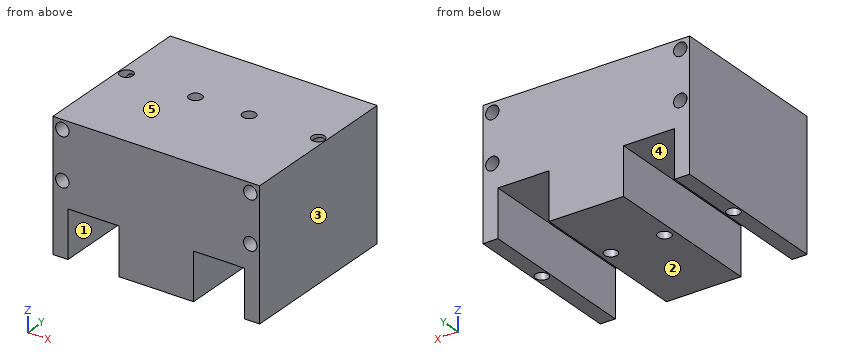
Autodesk Inventor part; units mm, degrees
ref_plane "YZ Plane" through (0, 0, 0) normal (1, 0, 0) x (0, 1, 0)
ref_plane "XZ Plane" through (0, 0, 0) normal (0, 1, 0) x (-1, 0, 0)
ref_plane "XY Plane" through (0, 0, 0) normal (0, 0, 1) x (1, 0, 0)
sketch "Esboço1" plane through (0, 0, 0) normal (0, 1, 0) x (-1, 0, 0)
  line L0 (0, 0) -> (-49.4, 0)
  line L1 (-49.4, 0) -> (-49.4, -15.9)
  line L2 (-49.4, -15.9) -> (0, -15.9)
  line L3 (0, -15.9) -> (0, 0)
  dimension "d0" = 49.4
  dimension "d1" = 15.9
extrude "Extrusão1" add sketch "Esboço1" along normal blind 40
sketch "Esboço2" plane through (0, 40, 0) normal (0, 1, 0) x (1, 0, 0)
  line L0 (49.4, 15.9) -> (0, 15.9)
  line L1 (0, 15.9) -> (4.5, 15.9)
  line L2 (4.5, 15.9) -> (4.5, 11.4)
  line L3 (4.5, 11.4) -> (0, 11.4)
  line L4 (0, 11.4) -> (0, 15.9)
  line L5 (0, 0) -> (49.4, 0)
  line L6 (0, 0) -> (4.5, 0)
  line L7 (4.5, 0) -> (4.5, 4.5)
  line L8 (4.5, 4.5) -> (0, 4.5)
  line L9 (0, 4.5) -> (0, 0)
  line L10 (49.4, 0) -> (49.4, 15.9)
  line L11 (49.4, 15.9) -> (44.9, 15.9)
  line L12 (44.9, 15.9) -> (44.9, 11.4)
  line L13 (44.9, 11.4) -> (49.4, 11.4)
  line L14 (49.4, 11.4) -> (49.4, 15.9)
  line L15 (49.4, 0) -> (44.9, 0)
  line L16 (44.9, 0) -> (44.9, 4.5)
  line L17 (44.9, 4.5) -> (49.4, 4.5)
  line L18 (49.4, 4.5) -> (49.4, 0)
  line L19 (2.25, 15.9) -> (2.25, 11.4)
  line L20 (2.25, 4.5) -> (2.25, 0)
  line L21 (47.15, 15.9) -> (47.15, 11.4)
  line L22 (47.15, 4.5) -> (47.15, 0)
  circle A0 centre (2.25, 13.65) radius 1.6
  circle A1 centre (2.25, 2.25) radius 1.6
  circle A2 centre (47.15, 13.65) radius 1.6
  circle A3 centre (47.15, 2.25) radius 1.6
  dimension "d4" = 4.5
  dimension "d5" = 4.5
  dimension "d6" = 4.5
  dimension "d7" = 4.5
  dimension "d8" = 4.5
  dimension "d9" = 4.5
  dimension "d10" = 4.5
  dimension "d11" = 4.5
  dimension "d12" = 3.2
  dimension "d13" = 3.2
  dimension "d14" = 3.2
  dimension "d15" = 3.2
extrude "Extrusão2" cut sketch "Esboço2" against normal blind 40 contours A2 L21 | L21 A2 | A3 L22 | L22 A3 | A0 L19 | L19 A0 | A1 L20 | L20 A1
sketch "Esboço3" plane through (49.4, 0, -15.9) normal (0, 0, -1) x (-1, 0, 0)
  line L0 (49.4, 40) -> (0, 40)
  line L1 (49.4, 0) -> (33.6, 0)
  line L2 (33.6, 0) -> (33.6, 40)
  line L3 (33.6, 40) -> (49.4, 40)
  line L4 (49.4, 40) -> (49.4, 0)
  line L5 (0, 0) -> (15.8, 0)
  line L6 (15.8, 0) -> (15.8, 40)
  line L7 (15.8, 40) -> (0, 40)
  line L8 (0, 40) -> (0, 0)
  line L9 (33.6, 0) -> (15.8, 0)
  line L10 (15.8, 0) -> (15.8, 40)
  line L11 (15.8, 40) -> (33.6, 40)
  line L12 (33.6, 40) -> (33.6, 0)
  line L13 (49.4, 0) -> (45.8, 0)
  line L14 (45.8, 0) -> (45.8, 40)
  line L15 (45.8, 40) -> (49.4, 40)
  line L16 (49.4, 40) -> (49.4, 0)
  line L17 (0, 0) -> (3.6, 0)
  line L18 (3.6, 0) -> (3.6, 40)
  line L19 (3.6, 40) -> (0, 40)
  line L20 (0, 40) -> (0, 0)
  point P0 (3.6, 0)
  point P1 (3.6, 40)
  dimension "d18" = 15.8
  dimension "d19" = 15.8
  dimension "d24" = 3.6
  dimension "d25" = 3.6
extrude "Extrusão3" add sketch "Esboço3" along normal blind 14.9 contours L2 L9 L6 L0
extrude "Extrusão4" add sketch "Esboço3" along normal blind 3.6 contours L4 L1 L14 L0 | L14 L1 L2 L0 | L6 L5 L18 L0 | L18 L5 L8 L0
extrude "Extrusão5" add sketch "Esboço3" along normal blind 14.9 contours L4 L1 L14 L0 | L18 L5 L8 L0
sketch "Esboço4" plane through (49.4, 0, -30.8) normal (0, 0, -1) x (-1, 0, 0)
  point P0 (49.4, 0)
sketch "Esboço5" plane through (49.4, 0, -30.8) normal (0, 0, -1) x (-1, 0, 0)
  line L0 (15.8, 40) -> (15.8, 0)
  line L1 (33.6, 0) -> (33.6, 40)
  line L2 (15.8, 40) -> (33.6, 40)
  line L3 (33.6, 40) -> (33.6, 20)
  line L4 (33.6, 20) -> (15.8, 20)
  line L5 (15.8, 20) -> (15.8, 40)
  line L6 (15.8, 20) -> (33.6, 20)
  line L7 (33.6, 20) -> (33.6, 0)
  line L8 (33.6, 0) -> (15.8, 0)
  line L9 (15.8, 0) -> (15.8, 20)
  line L10 (15.8, 20) -> (33.6, 20)
  line L11 (33.6, 20) -> (33.6, 25)
  line L12 (33.6, 25) -> (15.8, 25)
  line L13 (15.8, 25) -> (15.8, 20)
  line L14 (15.8, 20) -> (20.8, 20)
  line L15 (20.8, 20) -> (20.8, 25)
  line L16 (20.8, 25) -> (15.8, 25)
  line L17 (15.8, 25) -> (15.8, 20)
  line L18 (33.6, 20) -> (28.6, 20)
  line L19 (28.6, 20) -> (28.6, 25)
  line L20 (28.6, 25) -> (33.6, 25)
  line L21 (33.6, 25) -> (33.6, 20)
  line L22 (18.3, 25) -> (18.3, 20)
  circle A0 centre (18.3, 22.5) radius 1.55
  line L23 (31.1, 25) -> (31.1, 20)
  circle A1 centre (31.1, 22.5) radius 1.55
  line L24 (0, 40) -> (0, 0)
  line L25 (15.8, 25) -> (0, 25)
  line L26 (0, 25) -> (0, 20)
  line L27 (0, 20) -> (15.8, 20)
  line L28 (15.8, 20) -> (15.8, 25)
  line L29 (33.6, 25) -> (49.4, 25)
  line L30 (49.4, 25) -> (49.4, 20)
  line L31 (49.4, 20) -> (33.6, 20)
  line L32 (33.6, 20) -> (33.6, 25)
  line L33 (0, 22.5) -> (3.6, 22.5)
  line L34 (3.6, 40) -> (3.6, 0)
  line L35 (49.4, 22.5) -> (45.8, 22.5)
  line L36 (45.8, 0) -> (45.8, 40)
  circle A2 centre (1.8, 22.5) radius 1.55
  circle A3 centre (47.6, 22.5) radius 1.55
  point P0 (49.4, 0)
  dimension "d28" = 20
  dimension "d29" = 5
  dimension "d30" = 5
  dimension "d31" = 5
  dimension "d32" = 5
  dimension "d33" = 3.1
  dimension "d34" = 3.1
  dimension "d35" = 3.1
  dimension "d36" = 3.1
extrude "Extrusão6" cut sketch "Esboço5" against normal through all contours A0 L22 | L22 A0 | A2 L33 | L33 A2 | A1 L23 | L23 A1 | A3 L35 | L35 A3
Can you work these out from the model? Positions are in its coordinate system, mm. Face numbers are marked on the shaded views. A direction names the side the tool comes from. Coordinates: 2 decimals unless noted, no trailing zeros. Order: outer loops, then holes, each group sorted by start corner. A loop starts at its lowest first (then second) coordinate and runs counter-clockwise, first axis right, second up.
1. I'm going to push a flat-ended pin straight in: pin 1 (3.5 mm diameter, centred on x = 37.5, y = 20, fed in from -Z). Where does the tip first touch, or does it pass through?
2. If we section it at A-A (z = -25): Please give me the cut outline in (x, y).
3. Thinking about a two-plate mould opening in X: for the marked faces 3, 4 and 5, which applies, +X half, -X half, draft (parallel to the pull), parting line (faces both ways), or undercut?
4. I need wall thicknesses on line 1 (X direction, y = 25.5, z = -28); line 2 (Z direction, x = 2.25, y = 25); line 3 (X direction, y = 22.5, z = -11). Which ranges of each line are inside material? Lowest first, please.
5. If we section it at B-B (x = 31.1): Please give me the cut outline in (y, z), then the cut area to 3 significant figures.
6. For the marked faces 1 and 2, which set-ups out of +Z, -Z, +X, -X, +Y, -Y let a thin tool reach every point of the face, with its end or its side?
7. If we section it at D-D (z = -17.5): Please give me the cut outline in (x, y).
8. If we section it at C-C (y = 33.5): Please give me the cut outline in (x, z), then the cut area to 3 significant figures.
Entries:
1. pin 1: stops at z = -19.5
2. outline: (0, 0) - (3.6, 0) - (3.6, 40) - (0, 40) - close; (15.8, 0) - (33.6, 0) - (33.6, 40) - (15.8, 40) - close; (45.8, 0) - (49.4, 0) - (49.4, 40) - (45.8, 40) - close; hole circle Ø3.1 at (1.8, 22.5); hole circle Ø3.1 at (18.3, 22.5); hole circle Ø3.1 at (31.1, 22.5); hole circle Ø3.1 at (47.6, 22.5)
3. face 3: +X half
3. face 4: undercut
3. face 5: draft
4. line 1: x = 0 to 3.6, 15.8 to 33.6, 45.8 to 49.4
4. line 2: z = -30.8 to -15.25, -12.05 to -3.85, -0.65 to 0
4. line 3: x = 0 to 0.25, 3.35 to 16.75, 19.85 to 29.55, 32.65 to 46.05, 49.15 to 49.4
5. outline: (0, -30.8) - (20.95, -30.8) - (20.95, 0) - (0, 0) - close; (24.05, -30.8) - (40, -30.8) - (40, 0) - (24.05, 0) - close
5. area: 1,140 mm2
6. face 1: -Z, +Y, -Y
6. face 2: -Z, +X, -X, +Y, -Y
7. outline: (0, 0) - (49.4, 0) - (49.4, 40) - (0, 40) - close; hole circle Ø3.1 at (1.8, 22.5); hole circle Ø3.1 at (18.3, 22.5); hole circle Ø3.1 at (31.1, 22.5); hole circle Ø3.1 at (47.6, 22.5)
8. outline: (0, -30.8) - (3.6, -30.8) - (3.6, -19.5) - (15.8, -19.5) - (15.8, -30.8) - (33.6, -30.8) - (33.6, -19.5) - (45.8, -19.5) - (45.8, -30.8) - (49.4, -30.8) - (49.4, 0) - (0, 0) - close; hole circle Ø3.2 at (2.25, -13.65); hole circle Ø3.2 at (2.25, -2.25); hole circle Ø3.2 at (47.15, -13.65); hole circle Ø3.2 at (47.15, -2.25)
8. area: 1,210 mm2
